The drawing under review shows one solid part. Ordinate dimensions are in mm from its lowest x, y, z. A direction names the side the tool comes from. Give positions to 0.01 mm unless a question says otherwise; leave off trailing zeros. Order: outer loops, then holes, each group sorted by start corner. A loop starts at its lowest first (then second) coordinate and runs counter-clockwise, first axis right, second up. Notation, with made-up numbers: (-12, 88) -> (-8, 88) arc R34 cw to (-8, 119) -> close; hole circle Ø6 at (-3, 68.5). An arc over 180 degrees is marked (long way). One line per item, written item: value. Start each with the question number.
1) Consider section A-A (y = 59). State the section outline as (x, z) points, plus the area to 3 significant figures.
2) Tool access review of the marked faces 1 and 2: name each direction out of +Z, -Z, +X, -X, +Y, -Y from which nothing blocks a thin tool from reaching the whole face with its end or side.
3) For pin 1 (12 mm diameter, centred on x = 11.5, y = 63.5, fed in from -Z); pin 2 (0.8 mm diameter, centred on y = 65.5, z = 19, fed in from -X); pin 3 (3 mm diameter, centred on x = 18.5, y = 91.5, fed in from +Z); pin 4 (10 mm diameter, centred on y = 16.5, z = 9, fed in from +X), all flat-tipped, find the tip position at first contact; note any pin that passes through.
4) Wall thickness on line 1 along X through (y, z) = (105, 18); line 2 along Z through (x, y) = (19, 90); line 3 along Y through (x, z) = (28.5, 24): over which ranges is each line inside the solid? List them lowest first. Write a range as from..to.
5) Consider section B-B (y = 42). State the section outline as (x, z) points.
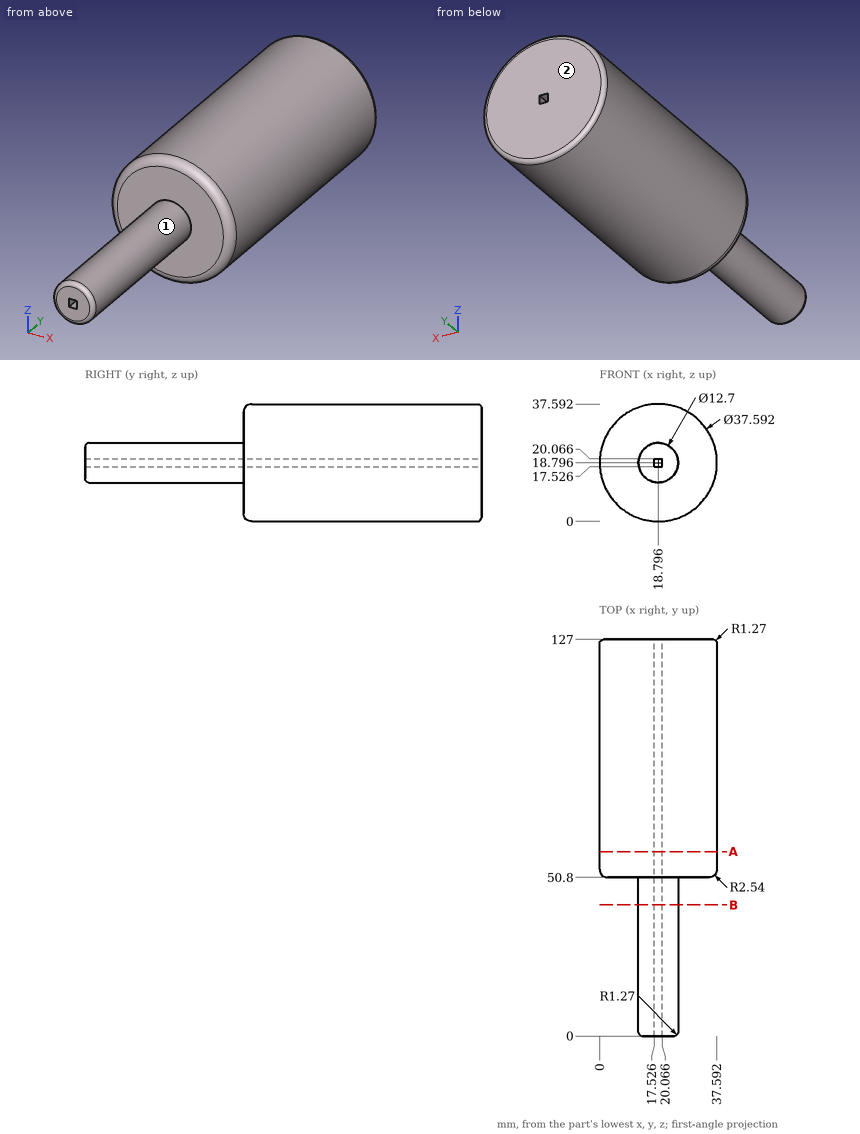
Checked values:
1. outline: circle Ø37.59 at (18.8, 18.8); hole (17.53, 17.53) -> (20.07, 17.53) -> (20.07, 20.07) -> (17.53, 20.07) -> close
1. area: 1,100 mm^2
2. face 1: -Y
2. face 2: +Z, -Z, +X, -X, +Y
3. pin 1: stops at z = 0.04
3. pin 2: stops at x = 0
3. pin 3: stops at z = 37.59
3. pin 4: stops at x = 22.96
4. line 1: x = 0.02..17.53, 20.07..37.58
4. line 2: z = 0..17.53, 20.07..37.59
4. line 3: y = 50.8..127
5. outline: circle Ø12.7 at (18.8, 18.8); hole (17.53, 17.53) -> (20.07, 17.53) -> (20.07, 20.07) -> (17.53, 20.07) -> close
